Check sheet for the modelled part. Datum: model origin and axes. Units: mm. Face numbers are marked on the shaded views. A direction names the side the tool comes from. Round coordinates to 2 decimals unless told otherwise and drop trailing zeros. Order: outer loops, then holes, each group sorted by start corner. A loop starts at its lowest first (then second) coordinate and runs counter-clockwise, first axis right, second up.
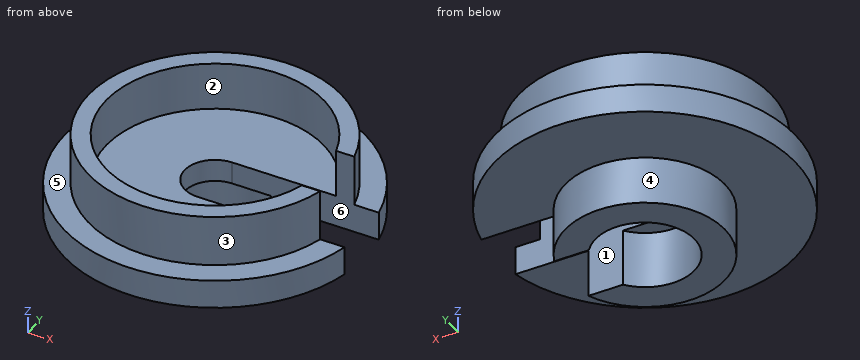
```python
from build123d import *

# Parameters (mm, degrees)
F3_DEPTH      = 21
F3_DEPTH_BACK = 5.081


# Not quite as in the source:
# - an extrude ends at something that could not be found from the text; its depth is read off the source's solid


with BuildPart() as f1:
    # F0 (on Front) → F1 (revolve)
    with BuildSketch(Plane.XZ):
        Polygon((1.9685, 2.286), (1.9685, 0), (3.175, 0), (3.175, 1.905), (5.969, 1.905), (5.969, 3.048), (5.0165, 3.048), (5.0165, 5.08), (4.318, 5.08), (4.318, 3.175), (1.2065, 3.175), (1.2065, 2.286), align=None)
    revolve(axis=Axis((0, 0, 1.6013546669), (0, 0, -1)))

    # F2 (on Top) → F3 (cut, two sides)
    with BuildSketch(Plane.XY) as f3_sk:
        with BuildLine():
            Line((5.845794963, 1.2065), (0, 1.2065))
            ThreePointArc((0, 1.2065), (-1.2065, 0), (0, -1.2065))
            Line((0, -1.2065), (5.845794963, -1.2065))
            ThreePointArc((5.845794963, -1.2065), (5.969, 0), (5.845794963, 1.2065))
        make_face()
    extrude(amount=-F3_DEPTH, mode=Mode.SUBTRACT)
    extrude(f3_sk.sketch, amount=F3_DEPTH_BACK, mode=Mode.SUBTRACT)


solid = f1.part
```
Item 1: Sectioned sample at B-B (x = -3.5). Record the cut outline in (y, z) (3 decimals).
Answer:
outline: (-4.835, 1.905) - (4.835, 1.905) - (4.835, 3.048) - (3.594, 3.048) - (3.594, 5.08) - (2.529, 5.08) - (2.529, 3.175) - (-2.529, 3.175) - (-2.529, 5.08) - (-3.594, 5.08) - (-3.594, 3.048) - (-4.835, 3.048) - close
Item 2: Scan lines: line 1 along Y through (x, z) = (0, 4.4); line 2 along Y through (x, z) = (0, 1.8) (1 decimal); line 3 along X through (y, z) = (0, 4.25). Record each from-to range of solid material in increasing order.
Answer:
line 1: y = -5.02 to -4.32, 4.32 to 5.02
line 2: y = -3.2 to -2, 2 to 3.2
line 3: x = -5.02 to -4.32
Item 3: Access from +Z, -Z, +X, -X, +Y, -Y to the whole of each face (thin tool, end or side, straight path). Record for the marked faces 4, 5 and 6.
Answer:
face 4: -Z
face 5: +Z
face 6: +Z, -Z, +X
Item 4: Go/stop test with flat-tipped pins: P1, Ø1.5, axis at x = 3.5, z = 2, coming from the +Y side; P2, Ø4.5, axis at x = 0, y = 0, coming from the +Z side (3 decimals); P3, Ø1.8, axis at x = 0, y = -0.5, coming from the -Z side. Record where each tip stops, or that it passes through.
Answer:
P1: stops at y = 5.3
P2: stops at z = 3.175
P3: stops at z = 2.29
Item 5: Release check for a two-part mould opening along X. For the marked faces 1, 2 and 3 record: released by +X, released by -X, zero draft, split by the parting line, or undercut.
Answer:
face 1: zero draft
face 2: undercut
face 3: split by the parting line
Item 6: Sectioned sample at A-A (y = 0). Record the cut outline in (x, z) (1 decimal).
Answer:
outline: (-6, 1.9) - (-3.2, 1.9) - (-3.2, 0) - (-2, 0) - (-2, 2.3) - (-1.2, 2.3) - (-1.2, 3.2) - (-4.3, 3.2) - (-4.3, 5.1) - (-5, 5.1) - (-5, 3) - (-6, 3) - close
Item 7: Sectioned sample at D-D (z = 3.75). Record the cut outline in (x, y), and give its area (3 significant figures).
Answer:
outline: (4.15, -1.21) arc R4.32 cw (long way) to (4.15, 1.21) - (4.87, 1.21) arc R5.02 ccw (long way) to (4.87, -1.21) - close
area: 18.8 mm2
